from build123d import *

# Parameters (mm, degrees)
F0_W     = 108.966
F0_H     = 28.956
F0_W_2   = 101.6
F0_H_2   = 22.86
F1_DEPTH = 2.54
F2_DEPTH = 2.54
F4_DEPTH = 2.032
F5_R     = 1.016


with BuildPart() as f1:
    # F0 (on Top) → F1 (new body)
    with BuildSketch(Plane.XY):
        Rectangle(F0_W, F0_H)
        Rectangle(F0_W_2, F0_H_2, mode=Mode.SUBTRACT)
        Rectangle(F0_W_2, F0_H_2)
    extrude(amount=F1_DEPTH)

    # F0 (on Top) → F2 (join)
    with BuildSketch(Plane.XY):
        Rectangle(F0_W_2, F0_H_2)
    extrude(amount=-F2_DEPTH)

    # F3 (on face) → F4 (join)
    with BuildSketch(Plane(origin=(0, 0, -2.54), x_dir=(1, 0, 0), z_dir=(0, 0, -1))):
        Polygon((-49.53, -6.6802), (-50.8, -6.6802), (-50.8, -11.43), (-46.0502, -11.43), (-46.0502, -10.16), (-49.53, -10.16), align=None)
        Polygon((50.8, 6.6802), (50.8, 11.43), (46.0502, 11.43), (46.0502, 10.16), (49.53, 10.16), (49.53, 6.6802), align=None)
        Polygon((50.8, -11.43), (50.8, -6.6802), (49.53, -6.6802), (49.53, -10.16), (46.0502, -10.16), (46.0502, -11.43), align=None)
        Polygon((-46.0502, 10.16), (-46.0502, 11.43), (-50.8, 11.43), (-50.8, 6.6802), (-49.53, 6.6802), (-49.53, 10.16), align=None)
    extrude(amount=F4_DEPTH)

    # F5
    f5_edges = [f1.edges().sort_by_distance(p)[0] for p in [
        (-50.8, -11.43, -2.286),
        (-50.8, 11.43, -2.286),
        (50.8, 11.43, -2.286),
        (50.8, -11.43, -2.286),
    ]]
    fillet(f5_edges, radius=F5_R)


solid = f1.part
Verification items for the finished model (mm, model axes). A direction names the side the tool comes from. Give positions to 0.01 mm unless a question says otherwise; leave off trailing zeros. Write each loop counter-clockwise with the first axis right and the second up, starting at its lowest first coordinate (ties: lowest second). Pieces come first, ordered by that corner, then holes. Notation, with made-up numbers: M 11.5,35.5 L 67.5,35.5 A28 cw 67.5,71.5 Z; hole C -19,38 d8. An arc over 180 degrees is marked long. Use CSV: the item, a comma, the result in double quotes.
1) Cross-section at C-C (y = -9.25). Enter the section's corners in (x, z).
Final values:
outline,"M -54.48,0 L -50.8,0 L -50.8,-4.57 L -49.53,-4.57 L -49.53,-2.54 L 49.53,-2.54 L 49.53,-4.57 L 50.8,-4.57 L 50.8,0 L 54.48,0 L 54.48,2.54 L -54.48,2.54 Z"
2) Access from +Z, -Z, +X, -X, +Y, -Y to the whole of each face (thin tool, end or side, straight path). Record for faces 1 (the face through (-1, -11.43, -1)), 2 (the face through (50.8, 0, -2)), 3 (the face through (48, -10.16, -4)).
Final values:
face 1,"-Z, +X, -X, -Y"
face 2,"-Z, +X, +Y, -Y"
face 3,"-Z"
3) Cross-section at B-B (x = 37). Enter the section's corners in (y, z).
Final values:
outline,"M -14.48,0 L -11.43,0 L -11.43,-2.54 L 11.43,-2.54 L 11.43,0 L 14.48,0 L 14.48,2.54 L -14.48,2.54 Z"
4) Material ranges on line 1 along X through (y, z) = (-10.5, -3.25); line 2 along Z through (x, y) = (-16.5, -12.25); line 3 along Z through (x, y) = (-6, 9.75), recorded low to high.
Final values:
line 1,"-50.8 to -46.05, 46.05 to 50.8"
line 2,"0 to 2.54"
line 3,"-2.54 to 2.54"
5) Go/stop test with flat-tipped pins: pin 1 Ø2 at (x, z) = (-47.5, -3.5) entering from -Y; pin 2 Ø1 at (y, z) = (10.5, -4) entering from +X; pin 3 Ø1.6 at (x, z) = (-47.5, -4) entering from +Y; pin 4 Ø4 at (y, z) = (8.5, -0.5) entering from +X. Record where each tip stops, or that it passes through.
Final values:
pin 1,"y = -11.43"
pin 2,"x = 50.8"
pin 3,"y = 11.43"
pin 4,"x = 54.48"
6) Cross-section at A-A (y = 2.5). Enter the section's corners in (x, z), plus the area to 3 significant figures.
Final values:
outline,"M -54.48,0 L -50.8,0 L -50.8,-2.54 L 50.8,-2.54 L 50.8,0 L 54.48,0 L 54.48,2.54 L -54.48,2.54 Z"
area,"535 mm²"
7) Release check for a two-part mould opening along X. For faces 4 (the face through (50, -10, -4.572)), 5 (the face through (-50.8, 0, -2)), 6 (the face through (-48, 10.16, -4)) record: released by +X, released by -X, zero draft, split by the parting line, or undercut.
Final values:
face 4,"zero draft"
face 5,"released by -X"
face 6,"undercut"
